Geometry check sheet. Reference: the model listing, model coordinates, mm. Face numbers are marked on the shaded views. Give positions to 0.01 mm unless a question says otherwise; leave off trailing zeros. Write each loop counter-clockwise with the first axis right and the second up, starting at its lowest first coordinate (ties: lowest second). Pieces come first, ordered by that corner, then holes.
(1) Cross-section at C-C (z = 5.2). Record the boundary of the cut face in (x, y).
(2) Thickness scan on line 1 along Y through (x, z) = (70, 3.15); line 2 along X through (y, z) = (59.25, 4.3); line 3 along Z through (x, y) = (73.5, 56.75). Record the ranges inside material, lowest first.
(3) Cross-section at A-A (y = 60). Record the boundary of the cut face in (x, z), and give its area (3 significant figures).
(4) Depth check by flat-ended pin: P1, Ø0.7, axis at y = 65, z = 4.5, coming from the +X side; P2, Ø1.2, axis at y = 55, z = 5.5, coming from the +X side. Enter the tip coordinate at first touch or a pass-through.
(5) Cross-section at B-B (x = 68). Record the boundary of the cut face in (y, z), and give its area (3 significant figures).
(6) Cross-section at D-D (z = 2.5). Record the boundary of the cut face in (x, y), and give its area (3 significant figures).
(7) Mould release check, pull along X, two halves, no side actions. Record for the marked faces 1, 2 and 3: +X half, -X half, draft (parallel to the pull), parting line (faces both ways), or undercut.
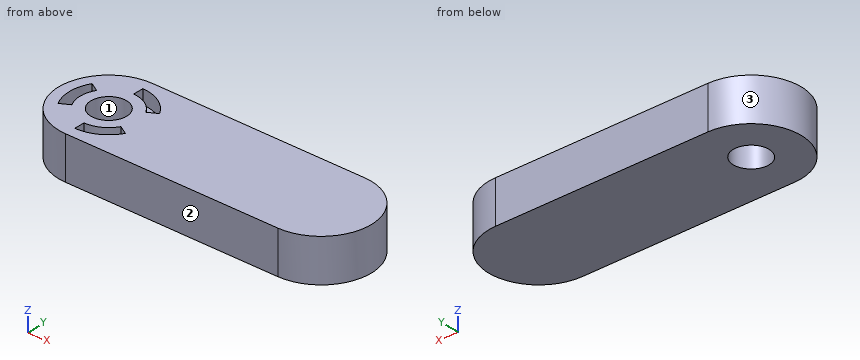
```python
from build123d import *

# Parameters (mm, degrees)
PAD008_DEPTH          = 6
SKETCH017_R           = 2.5
POCKET008_DEPTH       = 6.001
POCKET009_DEPTH       = 2
POLARPATTERN001_COUNT = 3


with BuildPart() as part:
    # Sketch016 → Pad008 (new body)
    with BuildSketch(Plane.XY):
        with BuildLine():
            ThreePointArc((0, 7), (-7, 0), (0, -7))
            Line((0, -7), (30, -7))
            ThreePointArc((30, -7), (37, 0), (30, 7))
            Line((0, 7), (30, 7))
        make_face()
    extrude(amount=PAD008_DEPTH)

    # Sketch017 (on Face6 of Pad008) → Pocket008 (cut, through all)
    with BuildSketch(Plane.XY.offset(6)):
        Circle(SKETCH017_R)
    extrude(amount=-POCKET008_DEPTH, mode=Mode.SUBTRACT)

    # Sketch019 (on Face5 of Pocket008) → Pocket009 (cut)
    with BuildSketch(Plane.XY.offset(6)):
        with BuildLine():
            ThreePointArc((-3.464102, 2), (-4, 0), (-3.464102, -2))
            Line((-4.76314, -2.75), (-3.464102, -2))
            ThreePointArc((-4.76314, 2.75), (-5.5, 0), (-4.76314, -2.75))
            Line((-4.76314, 2.75), (-3.464102, 2))
        make_face()
    pocket009 = extrude(amount=-POCKET009_DEPTH, mode=Mode.SUBTRACT)

    # PolarPattern001: Pocket009 ×3 about axis
    polarpattern001_axis = Axis((0, 0, 6), (0, 0, 1))
    for i in range(1, POLARPATTERN001_COUNT):
        add(pocket009.rotate(polarpattern001_axis, i * 360 / POLARPATTERN001_COUNT), mode=Mode.SUBTRACT)


with BuildPart() as part_1:
    # Body002 placement: moved
    add(part.part.moved(Location((70, 60, 0))))


solid = part_1.part
```
Reply:
1. outline: (70, 53) - (100, 53) arc R7 ccw to (100, 67) - (70, 67) arc R7 ccw to start; hole (65.24, 57.25) - (66.54, 58) arc R4 cw to (66.54, 62) - (65.24, 62.75) arc R5.5 ccw to start; hole circle Ø5 at (70, 60); hole (70, 54.5) arc R5.5 ccw to (74.76, 57.25) - (73.46, 58) arc R4 cw to (70, 56) - close; hole (70, 64) arc R4 cw to (73.46, 62) - (74.76, 62.75) arc R5.5 ccw to (70, 65.5) - close
2. line 1: y = 53 to 57.5, 62.5 to 67
2. line 2: x = 63.04 to 64.55, 66.07 to 67.62, 72.38 to 106.96
2. line 3: z = 0 to 4
3. outline: (63, 0) - (67.5, 0) - (67.5, 6) - (66, 6) - (66, 4) - (64.5, 4) - (64.5, 6) - (63, 6) - close; (72.5, 0) - (107, 0) - (107, 6) - (72.5, 6) - close
3. area: 231 mm2
4. P1: stops at x = 105.23
4. P2: stops at x = 105.44
5. outline: (53.29, 0) - (58.5, 0) - (58.5, 6) - (53.29, 6) - close; (61.5, 0) - (66.71, 0) - (66.71, 6) - (61.5, 6) - close
5. area: 62.5 mm2
6. outline: (70, 53) - (100, 53) arc R7 ccw to (100, 67) - (70, 67) arc R7 ccw to start; hole circle Ø5 at (70, 60)
6. area: 554 mm2
7. face 1: undercut
7. face 2: draft
7. face 3: -X half
